Input: part model. Units: mm. Frame: model coordinates. A direction names the side the tool comes from. Coordinates: 2 decimals unless noted, no trailing zeros. One line per question, with ' | ' between items. Start each with the question number.
```python
from build123d import *

# Parameters (mm, degrees)
SKETCH_1_W      = 200
SKETCH_1_H      = 200
SKETCH_1_R      = 2
EXTRUDE_2_DEPTH = 5


with BuildPart() as part:
    # 草图1 → 凸台-拉伸2 (new body)
    with BuildSketch(Plane(origin=(0, 0, 0), x_dir=(1, 0, 0), z_dir=(0, 1, 0))):
        Rectangle(SKETCH_1_W, SKETCH_1_H)
        with Locations(Location((-87, -87, 0), (0, 0, 270))):
            Circle(SKETCH_1_R, mode=Mode.SUBTRACT)
        with Locations(Location((-73, -87, 0), (0, 0, 270))):
            Circle(SKETCH_1_R, mode=Mode.SUBTRACT)
        with Locations(Location((-87, -73, 0), (0, 0, 270))):
            Circle(SKETCH_1_R, mode=Mode.SUBTRACT)
        with Locations(Location((-73, -73, 0), (0, 0, 270))):
            Circle(SKETCH_1_R, mode=Mode.SUBTRACT)
        with Locations(Location((-46.632517143, -20, 0), (0, 0, 270))):
            Circle(SKETCH_1_R, mode=Mode.SUBTRACT)
        with Locations(Location((-3.748020408, -35, 0), (0, 0, 270))):
            Circle(SKETCH_1_R, mode=Mode.SUBTRACT)
        with Locations(Location((73, -87, 0), (0, 0, 270))):
            Circle(SKETCH_1_R, mode=Mode.SUBTRACT)
        with Locations(Location((87, -87, 0), (0, 0, 270))):
            Circle(SKETCH_1_R, mode=Mode.SUBTRACT)
        with Locations(Location((73, -73, 0), (0, 0, 270))):
            Circle(SKETCH_1_R, mode=Mode.SUBTRACT)
        with Locations(Location((87, -73, 0), (0, 0, 270))):
            Circle(SKETCH_1_R, mode=Mode.SUBTRACT)
        with Locations(Location((31.251979592, -35, 0), (0, 0, 270))):
            Circle(SKETCH_1_R, mode=Mode.SUBTRACT)
        with Locations(Location((44.164957179, -20, 0), (0, 0, 270))):
            Circle(SKETCH_1_R, mode=Mode.SUBTRACT)
        with Locations(Location((64.164957179, -20, 0), (0, 0, 270))):
            Circle(SKETCH_1_R, mode=Mode.SUBTRACT)
        with BuildLine():
            Line((-79.805791506, 48), (-79.805791506, -48))
            ThreePointArc((-79.805791506, -48), (-79.708572332, -51.997635711), (-80, -48.009451568))
            Line((-80, -48.009451568), (-80, 48.009451568))
            ThreePointArc((-80, 48.009451568), (-79.708572332, 51.997635711), (-79.805791506, 48))
        make_face(mode=Mode.SUBTRACT)
        with Locations(Location((-46.632517143, 20, 0), (0, 0, 270))):
            Circle(SKETCH_1_R, mode=Mode.SUBTRACT)
        with Locations(Location((-3.748020408, 35, 0), (0, 0, 270))):
            Circle(SKETCH_1_R, mode=Mode.SUBTRACT)
        with Locations(Location((-87, 73, 0), (0, 0, 270))):
            Circle(SKETCH_1_R, mode=Mode.SUBTRACT)
        with Locations(Location((-73, 73, 0), (0, 0, 270))):
            Circle(SKETCH_1_R, mode=Mode.SUBTRACT)
        with Locations(Location((-87, 87, 0), (0, 0, 270))):
            Circle(SKETCH_1_R, mode=Mode.SUBTRACT)
        with Locations(Location((-73, 87, 0), (0, 0, 270))):
            Circle(SKETCH_1_R, mode=Mode.SUBTRACT)
        with Locations(Location((44.164957179, 20, 0), (0, 0, 270))):
            Circle(SKETCH_1_R, mode=Mode.SUBTRACT)
        with Locations(Location((31.251979592, 35, 0), (0, 0, 270))):
            Circle(SKETCH_1_R, mode=Mode.SUBTRACT)
        with Locations(Location((64.164957179, 20, 0), (0, 0, 270))):
            Circle(SKETCH_1_R, mode=Mode.SUBTRACT)
        with Locations(Location((73, 73, 0), (0, 0, 270))):
            Circle(SKETCH_1_R, mode=Mode.SUBTRACT)
        with Locations(Location((87, 73, 0), (0, 0, 270))):
            Circle(SKETCH_1_R, mode=Mode.SUBTRACT)
        with Locations(Location((73, 87, 0), (0, 0, 270))):
            Circle(SKETCH_1_R, mode=Mode.SUBTRACT)
        with Locations(Location((87, 87, 0), (0, 0, 270))):
            Circle(SKETCH_1_R, mode=Mode.SUBTRACT)
    extrude(amount=EXTRUDE_2_DEPTH)


solid = part.part
```
1) Ray query, line 1 (X direction, y = 3.2, z = -35); line 2 (X direction, y = 1.2, z = 73); line 3 (X direction, y = 1.8, z = -20). Return the intervals inside material, ascending.
2) First-contact query: P1, Ø3.5, axis at x = 64.16, z = -20, coming from the +Y side. Flat tip, straight axial feed; report the tip coordinate or a pass-through.
3) Access query for faces 1 (the face through (-100, 2, 1)), 2 (the face through (-80, 2, 1)). Directions: +Z, -Z, +X, -X, +Y, -Y. A direction counts if a zero-diameter tool reaches every point of the face in a straight line with its end or side. Return the directions, or none.
Answer block:
1) line 1: x = -100 to -80, -79.81 to -5.75, -1.75 to 29.25, 33.25 to 100 | line 2: x = -100 to -89, -85 to -75, -71 to 71, 75 to 85, 89 to 100 | line 3: x = -100 to -80, -79.81 to -48.63, -44.63 to 42.16, 46.16 to 62.16, 66.16 to 100
2) P1: passes through
3) face 1: +Z, -Z, -X, +Y, -Y | face 2: +Y, -Y
